```python
from build123d import *

# Parameters (mm, degrees)
BOSS_EXTRUDE1_DEPTH = 6.05


with BuildPart() as part:
    # Sketch1 → Boss-Extrude1 (new body)
    with BuildSketch(Plane.YZ):
        with BuildLine():
            Line((-125, 7.125), (125, 7.125))
            ThreePointArc((125, 7.125), (132.125, 0), (125, -7.125))
            Line((125, -7.125), (-125, -7.125))
            ThreePointArc((-125, -7.125), (-132.125, 0), (-125, 7.125))
        make_face()
        with BuildLine():
            Line((-125, 6.125), (125, 6.125))
            ThreePointArc((125, 6.125), (131.125, 0), (125, -6.125))
            Line((125, -6.125), (-125, -6.125))
            ThreePointArc((-125, -6.125), (-131.125, 0), (-125, 6.125))
        make_face(mode=Mode.SUBTRACT)
    extrude(amount=BOSS_EXTRUDE1_DEPTH)


solid = part.part
```
Here's how the part is built. I have some questions about the finished solid (model axes, mm). A direction names the side the tool comes from. Round coordinates to 2 decimals unless told otherwise and drop trailing zeros. Loops run counter-clockwise (first coordinate to the right, second up) from the corner with the lowest first, then second, coordinate; pieces in that order, holes last. Notation, with made-up numbers: (29, 72.5) -> (41, 72.5) arc R28 ccw to (41, 97.5) -> close; hole circle Ø5 at (-34.75, 61). An arc over 180 degrees is marked (long way). Answer as CSV lines item,"result". Start each with the question number.
1. For faces 4 (the face through (2.983, -132.123, -0.157)), 5 (the face through (2.983, 131.124, 0.135)), which set-ups out of +Z, -Z, +X, -X, +Y, -Y let a thin tool reach every point of the face, with its end or its side?
2. Imagine slicing it at B-B on z = 0. Write out the boundary of the cut face in (x, y) (3 decimals), plus the area to 3 significant figures.
3. I'm going to push flat-ended pins straight in: P1, Ø2, axis at x = 2, z = -2.5, coming from the -Y side; P2, Ø3, axis at x = 2.5, z = 3.5, coming from the +Y side. Where does each tip first touch, or does it pass through?
4. Imagine slicing it at A-A on y = 113. Write out the boundary of the cut face in (x, z) (3 decimals).
5. I need wall thicknesses on probe 1 along Z at (x, y) = (3, 101.5) (3 decimals); probe 2 along Y at (x, z) = (3, -0.5); probe 3 along Y at (x, z) = (4.25, -1). Which ranges of each line are inside material? Lowest first, please. Write a range as from..to.
6. Imagine slicing it at C-C on x = 1.75. Write out the boundary of the cut face in (y, z) (3 decimals).
7. If we mould it in two halves opening along Y, with no side actions, what happens to faces 1 (the face through (2.983, 132.123, 0.157)), 2 (the face through (6.05, 0.6, 6.4)), 3 (the face through (3, 2, -6.125))? For each: pulls with the +Y half, pulls with the -Y half, needs draft (parallel to the pull), parting line crosses it, or undercut.
Solution:
1,face 4,"+X, -X, -Y"
1,face 5,"+X, -X"
2,outline,"(0, -132.125) -> (6.05, -132.125) -> (6.05, -131.125) -> (0, -131.125) -> close; (0, 131.125) -> (6.05, 131.125) -> (6.05, 132.125) -> (0, 132.125) -> close"
2,area,"12.1 mm²"
3,P1,"y = -131.97"
3,P2,"y = 131.84"
4,outline,"(0, -7.125) -> (6.05, -7.125) -> (6.05, -6.125) -> (0, -6.125) -> close; (0, 6.125) -> (6.05, 6.125) -> (6.05, 7.125) -> (0, 7.125) -> close"
5,probe 1,"-7.125..-6.125, 6.125..7.125"
5,probe 2,"-132.11..-131.1, 131.1..132.11"
5,probe 3,"-132.05..-131.04, 131.04..132.05"
6,outline,"(-125, -7.125) -> (125, -7.125) arc R7.125 ccw to (125, 7.125) -> (-125, 7.125) arc R7.125 ccw to start; hole (-125, -6.125) -> (125, -6.125) arc R6.125 ccw to (125, 6.125) -> (-125, 6.125) arc R6.125 ccw to start"
7,face 1,"pulls with the +Y half"
7,face 2,"needs draft"
7,face 3,"undercut"
